Work out the finished part from the listing and answer in its coordinate system (mm). Coordinates: 2 decimals unless noted, no trailing zeros. Order: outer loops, then holes, each group sorted by start corner. A loop starts at its lowest first (then second) coordinate and runs counter-clockwise, first axis right, second up. Notation, with made-up numbers: M 19.25,7 L 41.25,7 A34 cw 41.25,41 Z; hole C 76,63.25 d2. An arc over 180 degrees is marked long. Use a Markdown table: item, result.
from build123d import *

# Parameters (mm, degrees)
BOSS_EXTRUDE1_DEPTH = 2


with BuildPart() as part:
    # Sketch1 → Boss-Extrude1 (new body)
    with BuildSketch(Plane.XY):
        with BuildLine():
            Line((0, -3), (25, -3))
            Line((25, -3), (25, -17))
            ThreePointArc((25, -17), (25.878679656, -19.121320344), (28, -20))
            Line((28, -20), (50, -20))
            Line((50, -20), (50, 40))
            Line((50, 40), (-50, 40))
            Line((-50, 40), (-50, -3))
            Line((-50, -3), (-25, -3))
            Line((-25, -3), (-25, -17))
            ThreePointArc((-25, -17), (-24.121320344, -19.121320344), (-22, -20))
            Line((-22, -20), (-3, -20))
            ThreePointArc((-3, -20), (-0.878679656, -19.121320344), (0, -17))
            Line((0, -17), (0, -3))
        make_face()
    extrude(amount=BOSS_EXTRUDE1_DEPTH)


solid = part.part
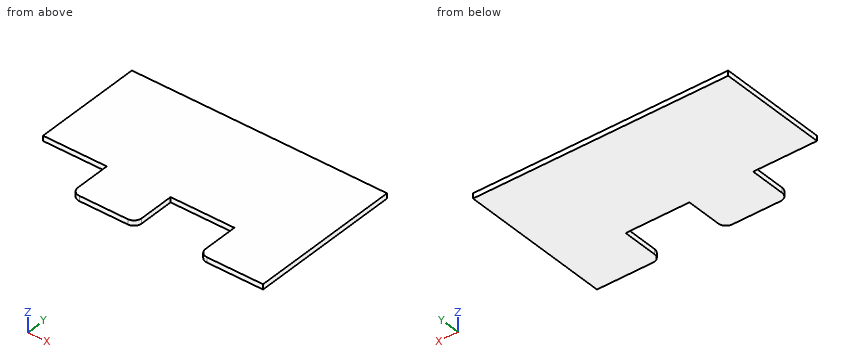
(1) A cutting plane is placed at B-B (z = 0.65). Determine the outline of the cut face in (x, y), then the cut area to 3 significant figures.
Conclusion:
| item | result |
|---|---|
| outline | M -50,-3 L -25,-3 L -25,-17 A3 ccw -22,-20 L -3,-20 A3 ccw 0,-17 L 0,-3 L 25,-3 L 25,-17 A3 ccw 28,-20 L 50,-20 L 50,40 L -50,40 Z |
| area | 5,140 mm2 |
(2) A cutting plane is placed at A-A (y = -14). Determine the outline of the cut face in (x, z), then the cut area to 3 significant figures.
Conclusion:
| item | result |
|---|---|
| outline | M -25,0 L 0,0 L 0,2 L -25,2 Z; M 25,0 L 50,0 L 50,2 L 25,2 Z |
| area | 100 mm2 |
(3) Given P1, Ø1, axis at x = 7, z = 1.5, coming from the -Y side; P2, Ø0.6, axis at y = -7, z = 1, coming from the -X side, each flat-ended and moving along its own axis, determine where each tip first touches the part or whether it passes through.
Conclusion:
| item | result |
|---|---|
| P1 | y = -3 |
| P2 | x = -25 |
(4) A cutting plane is placed at C-C (x = -27.5). Determine the outline of the cut face in (y, z).
Conclusion:
| item | result |
|---|---|
| outline | M -3,0 L 40,0 L 40,2 L -3,2 Z |
(5) Straight lines are drawn through the part: L1, parallel to X at y = -12, z = 0.8; L2, parallel to Y at x = 18.5, z = 0.5. For each, find the intervals that lie inside material, in ascending order.
Conclusion:
| item | result |
|---|---|
| L1 | -25 to 0, 25 to 50 |
| L2 | -3 to 40 |
